Could you check a few things on this model? Use its own coordinates, in mm. A direction names the side the tool comes from. Round coordinates to 2 decimals unless told otherwise and drop trailing zeros. Loops run counter-clockwise (first coordinate to the right, second up) from the corner with the lowest first, then second, coordinate; pieces in that order, holes last. Notation, with made-up numbers: (-7, 13.25) -> (36, 13.25) arc R31 ccw to (36, 37.25) -> close; hole circle Ø3 at (75, 49.25). An arc over 180 degrees is marked (long way). Put each result on its own line as item: value. Start each with the question number.
1. Which directions (+Z, -Z, +X, -X, +Y, -Y) give clear straight access to the entire face, cutting with the end or side of a thin tool? Please do faces 1 (the flat face through (-5, 19.5, -1)), 2 (the cylindrical face through (-2.89, 9.61, -3.77)), 3 (the cylindrical face through (-5.75, -5.423, 1.273)).
2. Imagine slicing it at D-D, the plane y = 5. Please give me the cut outline in (x, z), and give its area (3 significant figures).
3. I'm going to push flat-ended pins straight in: P1, Ø4, axis at y = -6.5, z = 0, coming from the +X side; P2, Ø2, axis at x = -2.5, y = 0, coming from the +Z side; P3, Ø3, axis at y = -3.5, z = -3, coming from the -X side; P4, Ø6, axis at x = -1.5, z = 1.5, coming from the -Y side. Where does each tip first touch, or does it pass through?
4. Imagine slicing it at A-A, the plane x = 0. Please give me the cut outline in (y, z).
5. Imagine slicing it at C-C, the plane y = -2. Count the separate pieces of the cut face and the enclosed holes in it, and give its area (3 significant figures).
6. Imagine slicing it at B-B, the plane z = 0. Please give me the cut outline in (x, y).
7. I need wall thicknesses on line 1 (X direction, y = 15, z = 0); line 2 (X direction, y = -9, z = 1) (3 decimals); line 3 (Y direction, x = -4.75, z = -3.75). Which ranges of each line are inside material? Lowest first, please. Write a range as [from, to].
8. If we mould it in two halves opening along X, with no side actions, what happens to faces 4 (the cylindrical face through (4.95, -5.42, 0.6)), 5 (the cylindrical face through (1.9, 9.6, 5.9)), 6 (the flat face through (-5.6, -11, 0.9))? For each: pulls with the +X half, pulls with the -X half, needs draft (parallel to the pull), parting line crosses it, or undercut.
```python
from build123d import *

# Parameters (mm, degrees)
SKETCH1_R               = 6.2
BOSS_EXTRUDE1_DEPTH     = 19.5
SKETCH2_R               = 2
BOSS_EXTRUDE2_DEPTH     = 2.8
SKETCH3_R               = 0.4
BOSS_EXTRUDE4_DEPTH     = 3.5
CUT_EXTRUDE1_START      = -0.2
SKETCH4_R               = 4.75
SKETCH4_R_2             = 2
CUT_EXTRUDE1_DEPTH      = 0.2
SKETCH5_R               = 0.4
BOSS_EXTRUDE5_DEPTH     = 11
CUT_EXTRUDE3_DEPTH      = 32.543145056
CUT_EXTRUDE3_DEPTH_BACK = 19.3
SKETCH6_R               = 4.75


with BuildPart() as part:
    # Sketch1 → Boss-Extrude1 (new body)
    with BuildSketch(Plane(origin=(0, 0, 0), x_dir=(1, 0, 0), z_dir=(0, 1, 0))):
        with Locations(Location((0, 0, 0), (0, 0, 270))):
            Circle(SKETCH1_R)
    extrude(amount=BOSS_EXTRUDE1_DEPTH)

    # Sketch2 → Boss-Extrude2 (add)
    with BuildSketch(Plane(origin=(0, 19.5, 0), x_dir=(1, 0, 0), z_dir=(0, 1, 0))):
        with Locations(Location((0, 0, 0), (0, 0, 270))):
            Circle(SKETCH2_R)
    extrude(amount=BOSS_EXTRUDE2_DEPTH)

    # Sketch3 → Boss-Extrude4 (add)
    with BuildSketch(Plane(origin=(0, 22.3, 0), x_dir=(1, 0, 0), z_dir=(0, 1, 0))):
        with Locations(Location((-0.41145274, -0.237271907, 0), (0, 0, 270))):
            Circle(SKETCH3_R)
        with Locations(Location((-0.09128588, 1.346231062, 0), (0, 0, 270))):
            Circle(SKETCH3_R)
        with Locations(Location((0.706061251, 1.146478436, 0), (0, 0, 270))):
            Circle(SKETCH3_R)
        with Locations(Location((1.233716983, 0.516206281, 0), (0, 0, 270))):
            Circle(SKETCH3_R)
        with Locations(Location((1.29013476, -0.30384286, 0), (0, 0, 270))):
            Circle(SKETCH3_R)
        with Locations(Location((0.853764908, -1.000438089, 0), (0, 0, 270))):
            Circle(SKETCH3_R)
        with Locations(Location((0.09128588, -1.307503705, 0), (0, 0, 270))):
            Circle(SKETCH3_R)
        with Locations(Location((-0.706061251, -1.107751078, 0), (0, 0, 270))):
            Circle(SKETCH3_R)
        with Locations(Location((-1.233716983, -0.477478923, 0), (0, 0, 270))):
            Circle(SKETCH3_R)
        with Locations(Location((-1.29013476, 0.342570218, 0), (0, 0, 270))):
            Circle(SKETCH3_R)
        with Locations(Location((-0.853764908, 1.039165447, 0), (0, 0, 270))):
            Circle(SKETCH3_R)
        with Locations(Location((0, 0.516206281, 0), (0, 0, 270))):
            Circle(SKETCH3_R)
        with Locations(Location((0.441742202, -0.237271907, 0), (0, 0, 270))):
            Circle(SKETCH3_R)
    extrude(amount=BOSS_EXTRUDE4_DEPTH)

    # Sketch4 → Cut-Extrude1 (cut)
    with BuildSketch(Plane(origin=(0, 19.5, 0), x_dir=(1, 0, 0), z_dir=(0, 1, 0)).offset(CUT_EXTRUDE1_START)):
        with Locations(Location((0, 0, 0), (0, 0, 270))):
            Circle(SKETCH4_R)
        with Locations(Location((0, 0, 0), (0, 0, 270))):
            Circle(SKETCH4_R_2, mode=Mode.SUBTRACT)
    extrude(amount=CUT_EXTRUDE1_DEPTH, mode=Mode.SUBTRACT)

    # Sketch5 → Boss-Extrude5 (add)
    with BuildSketch(Plane.XZ):
        with Locations(Location((-5.700120356, 0, 0), (0, 0, 90))):
            Circle(SKETCH5_R)
        with Locations(Location((-5.629942415, 0.891695278, 0), (0, 0, 90))):
            Circle(SKETCH5_R)
        with Locations(Location((-4.791405516, 0, 0), (0, 0, 90))):
            Circle(SKETCH5_R)
        with Locations(Location((-4.703373902, 0.914243273, 0), (0, 0, 90))):
            Circle(SKETCH5_R)
        with Locations(Location((-4.703373902, -0.914243273, 0), (0, 0, 90))):
            Circle(SKETCH5_R)
        with Locations(Location((-5.629942415, -0.891695278, 0), (0, 0, 90))):
            Circle(SKETCH5_R)
        with Locations(Location((5.629942415, -0.891695278, 0), (0, 0, 90))):
            Circle(SKETCH5_R)
        with Locations(Location((4.703373902, -0.914243273, 0), (0, 0, 90))):
            Circle(SKETCH5_R)
        with Locations(Location((4.703373902, 0.914243273, 0), (0, 0, 90))):
            Circle(SKETCH5_R)
        with Locations(Location((4.791405516, 0, 0), (0, 0, 90))):
            Circle(SKETCH5_R)
        with Locations(Location((5.629942415, 0.891695278, 0), (0, 0, 90))):
            Circle(SKETCH5_R)
        with Locations(Location((5.700120356, 0, 0), (0, 0, 90))):
            Circle(SKETCH5_R)
    extrude(amount=BOSS_EXTRUDE5_DEPTH)

    # Sketch6 → Cut-Extrude3 (cut, two sides: drawn at the far end of the back side and taken through both)
    with BuildSketch(Plane(origin=(0, 19.3, 0), x_dir=(1, 0, 0), z_dir=(0, 1, 0)).offset(-CUT_EXTRUDE3_DEPTH_BACK)):
        with Locations(Location((0, 0, 0), (0, 0, 270))):
            Circle(SKETCH6_R)
    extrude(amount=CUT_EXTRUDE3_DEPTH + CUT_EXTRUDE3_DEPTH_BACK, mode=Mode.SUBTRACT)


solid = part.part
```
Entries:
1. face 1: +Z, -Z, +X, -X, +Y
1. face 2: +Y
1. face 3: -Y
2. outline: circle Ø12.4 at (0, 0); hole circle Ø9.5 at (0, 0)
2. area: 49.9 mm^2
3. P1: x = 6.1
3. P2: z = 6.02
3. P3: through
3. P4: y = -11
4. outline: (0, -6.2) -> (19.5, -6.2) -> (19.5, -4.75) -> (0, -4.75) -> close; (0, 4.75) -> (19.5, 4.75) -> (19.5, 6.2) -> (0, 6.2) -> close
5. separate pieces: 12
5. enclosed holes: 0
5. area: 6.03 mm^2
6. outline: (-6.2, 0) -> (-6.1, 0) -> (-6.1, -11) -> (-5.3, -11) -> (-5.3, 0) -> (-5.19, 0) -> (-5.19, -11) -> (-4.39, -11) -> (-4.39, 0) -> (-4.75, 0) -> (-4.75, 19.5) -> (-6.2, 19.5) -> close; (4.39, -11) -> (5.19, -11) -> (5.19, 0) -> (5.3, 0) -> (5.3, -11) -> (6.1, -11) -> (6.1, 0) -> (6.2, 0) -> (6.2, 19.5) -> (4.75, 19.5) -> (4.75, 0) -> (4.39, 0) -> close
7. line 1: [-6.2, -4.75], [4.75, 6.2]
7. line 2: [-6.015, -5.245], [-5.094, -4.313], [4.313, 5.094], [5.245, 6.015]
7. line 3: [0, 19.5]
8. face 4: undercut
8. face 5: parting line crosses it
8. face 6: needs draft
